```python
from build123d import *

# Parameters (mm, degrees)
SKETCH5_W               = 175.26
SKETCH5_H               = 137.414
SKETCH5_W_2             = 165.1
SKETCH5_H_2             = 127.254
BOSS_EXTRUDE2_DEPTH     = 43.18
SKETCH7_W               = 175.26
SKETCH7_H               = 137.414
BOSS_EXTRUDE4_DEPTH     = 10.16
SKETCH9_W               = 127.254
SKETCH9_H               = 2.159
CUT_EXTRUDE1_DEPTH      = 8.128
CUT_EXTRUDE2_DEPTH      = 13.208
CUT_EXTRUDE2_DEPTH_BACK = 147.066
SKETCH11_W              = 88.9
SKETCH11_H              = 33.02
CUT_EXTRUDE3_DEPTH      = 10.16
SKETCH12_W              = 25.4
SKETCH12_H              = 25.4
BOSS_EXTRUDE5_DEPTH     = 76.2
SKETCH13_W              = 20.32
SKETCH13_H              = 20.32
CUT_EXTRUDE4_DEPTH      = 76.2
SKETCH14_R              = 2.54
BOSS_EXTRUDE6_DEPTH     = 7.62
SKETCH15_R              = 2.54
BOSS_EXTRUDE7_DEPTH     = 25.4


with BuildPart() as part:
    # Sketch5 → Boss-Extrude2 (new body)
    with BuildSketch(Plane(origin=(0, 0, 0), x_dir=(1, 0, 0), z_dir=(0, 1, 0))):
        with Locations((82.55, 63.627)):
            Rectangle(SKETCH5_W, SKETCH5_H)
        with Locations((82.55, 63.627)):
            Rectangle(SKETCH5_W_2, SKETCH5_H_2, mode=Mode.SUBTRACT)
    extrude(amount=BOSS_EXTRUDE2_DEPTH)

    # Sketch7 → Boss-Extrude4 (add)
    with BuildSketch(Plane(origin=(0, 0, 0), x_dir=(1, 0, 0), z_dir=(0, 1, 0))):
        with Locations((82.55, 63.627)):
            Rectangle(SKETCH7_W, SKETCH7_H)
    extrude(amount=-BOSS_EXTRUDE4_DEPTH)

    # Sketch9 → Cut-Extrude1 (cut)
    with BuildSketch(Plane(origin=(170.18, 0, 0), x_dir=(0, 0, -1), z_dir=(1, 0, 0))):
        with Locations((63.627, 1.0795)):
            Rectangle(SKETCH9_W, SKETCH9_H)
    extrude(amount=-CUT_EXTRUDE1_DEPTH, mode=Mode.SUBTRACT)

    # Sketch10 → Cut-Extrude2 (cut, two sides: drawn at the far end of the back side and taken through both)
    with BuildSketch(Plane.XY.offset(5.08).offset(-CUT_EXTRUDE2_DEPTH_BACK)):
        with BuildLine():
            Line((69.85, 43.18), (95.25, 43.18))
            Line((95.25, 43.18), (95.25, 7.62))
            ThreePointArc((95.25, 7.62), (93.018153673, 2.231846327), (87.63, 0))
            Line((87.63, 0), (77.47, 0))
            ThreePointArc((77.47, 0), (72.081846327, 2.231846327), (69.85, 7.62))
            Line((69.85, 7.62), (69.85, 43.18))
        make_face()
    extrude(amount=CUT_EXTRUDE2_DEPTH + CUT_EXTRUDE2_DEPTH_BACK, mode=Mode.SUBTRACT)

    # Sketch11 → Cut-Extrude3 (cut)
    with BuildSketch(Plane.XZ.offset(10.16)):
        with Locations((82.55, -63.627)):
            Rectangle(SKETCH11_W, SKETCH11_H)
    extrude(amount=-CUT_EXTRUDE3_DEPTH, mode=Mode.SUBTRACT)

    # Sketch12 → Boss-Extrude5 (add)
    with BuildSketch(Plane.XZ.offset(10.16)):
        with Locations((7.62, -7.62)):
            Rectangle(SKETCH12_W, SKETCH12_H)
        with Locations((157.48, -7.62)):
            Rectangle(SKETCH12_W, SKETCH12_H)
        with Locations((157.48, -119.634)):
            Rectangle(SKETCH12_W, SKETCH12_H)
        with Locations((7.62, -119.634)):
            Rectangle(SKETCH12_W, SKETCH12_H)
    extrude(amount=BOSS_EXTRUDE5_DEPTH)

    # Sketch13 → Cut-Extrude4 (cut)
    with BuildSketch(Plane.XZ.offset(86.36)):
        with Locations((7.62, -7.62)):
            Rectangle(SKETCH13_W, SKETCH13_H)
        with Locations((157.48, -7.62)):
            Rectangle(SKETCH13_W, SKETCH13_H)
        with Locations((157.48, -119.634)):
            Rectangle(SKETCH13_W, SKETCH13_H)
        with Locations((7.62, -119.634)):
            Rectangle(SKETCH13_W, SKETCH13_H)
    extrude(amount=-CUT_EXTRUDE4_DEPTH, mode=Mode.SUBTRACT)

    # Sketch14 → Boss-Extrude6 (add)
    with BuildSketch(Plane.XY.offset(5.08)):
        with BuildLine():
            Line((69.409163099, -10.16), (69.409163099, -35.56))
            ThreePointArc((69.409163099, -35.56), (82.55, -48.700836901), (95.690836901, -35.56))
            Line((95.690836901, -35.56), (95.690836901, -10.16))
            Line((95.690836901, -10.16), (69.409163099, -10.16))
        make_face()
        with Locations((82.55, -35.56)):
            Circle(SKETCH14_R, mode=Mode.SUBTRACT)
    boss_extrude6 = extrude(amount=-BOSS_EXTRUDE6_DEPTH)

    # Mirror2: Boss-Extrude6 across plane
    add(boss_extrude6.mirror(Plane.XY.offset(-63.627)))

    # Sketch15 → Boss-Extrude7 (add)
    with BuildSketch(Plane(origin=(0, 0, -132.334), x_dir=(-1, 0, 0), z_dir=(0, 0, -1))):
        with Locations(Location((-122.428, 13.97, 0), (0, 0, 180))):
            Circle(SKETCH15_R)
    extrude(amount=BOSS_EXTRUDE7_DEPTH)


solid = part.part
```
CAD build for the part. Positions are in the model's coordinates, mm. A direction names the side the tool comes from. Coordinates: 2 decimals unless noted, no trailing zeros. Write each loop counter-clockwise with the first axis right and the second up, starting at its lowest first coordinate (ties: lowest second). Pieces come first, ordered by that corner, then holes. Notation, with made-up numbers: (4.5, -15.75) -> (60.5, -15.75) arc R34 ccw to (60.5, 17.25) -> close; hole circle Ø7 at (69.5, -29). An arc over 180 degrees is marked (long way). Return JSON: item names as keys, results as strings. Group by question number.
Q1. Flat gauge pins, fed straight in: pin 1 (10 mm diameter, centred on x = 156, y = -49, fed in from -Z); pin 2 (12 mm diameter, centred on x = 61.5, z = -86, fed in from +Y); pin 3 (10 mm diameter, centred on x = 11.5, z = -123.5, fed in from -Y). Where does each tip first touch, or does it go through?
Q2. Cut at A-A, the plane y = -65. State how many separate pieces and enclosed holes the cut face has, then the cut area to 3 significant figures.
Q3. Drill centre lines: line 1 (X direction, y = -79, z = -10); line 2 (Z direction, x = 4.5, y = -57.5); line 3 (X direction, y = 10, z = -11.5). Where is each one in solid material? Low to high.
Q4. Cut at B-B, the plane x = 64. Give the cut face in (y, z), then the cut area to 3 significant figures.
Q5. Pull direction Z, two halves, no side cores. Call faces 1 (the face through (146, -86.36, -7)), 2 (the face through (7, -48, -106.934)): released by +Z, released by -Z, zero draft, split by the parting line, or undercut.
Q6. Cut at D-D, the plane z = -99. Give the cut face in (x, y), then the cut area to 3 significant figures.
Q7. Which spindle directions (+Z, -Z, +X, -X, +Y, -Y) get a long thin tool onto all of the face, cutting with end or side? Do faces 3 (the face through (157, -10.16, -119)), 4 (the face through (72.141, 2.173, 2.504)), 5 (the face through (168, 2.159, -63)), 6 (the face through (20.32, -48, -8)), 7 (the face through (127, -5, -64)). Say none if no direction does.
Q8. Cut at C-C, the plane y = 13.97. Give the cut face in (x, z), then the cut area to 3 significant figures.
Returned:
{
 "1": {"pin 1": "stops at z = -132.33", "pin 2": "stops at y = 0", "pin 3": "stops at y = -10.16"},
 "2": {"separate pieces": "4", "enclosed holes": "4", "area": "929 mm2"},
 "3": {"line 1": "x = -5.08 to -2.54, 17.78 to 20.32, 144.78 to 147.32, 167.64 to 170.18", "line 2": "z = -132.33 to -129.79, -109.47 to -106.93, -20.32 to -17.78, 2.54 to 5.08", "line 3": "x = -5.08 to 0, 165.1 to 170.18"},
 "4": {"outline": "(-10.16, -132.33) -> (43.18, -132.33) -> (43.18, -127.25) -> (0, -127.25) -> (0, -80.14) -> (-10.16, -80.14) -> close; (-10.16, -47.12) -> (0, -47.12) -> (0, 0) -> (43.18, 0) -> (43.18, 5.08) -> (-10.16, 5.08) -> close", "area": "1,500 mm2"},
 "5": {"face 1": "zero draft", "face 2": "undercut"},
 "6": {"outline": "(-5.08, -10.16) -> (170.18, -10.16) -> (170.18, 0) -> (0, 0) -> (0, 43.18) -> (-5.08, 43.18) -> close; (165.1, 2.16) -> (170.18, 2.16) -> (170.18, 43.18) -> (165.1, 43.18) -> close", "area": "2,210 mm2"},
 "7": {"face 3": "-Y", "face 4": "+Z, -Z, +Y", "face 5": "+X", "face 6": "+Z, -Z, -Y", "face 7": "+Y, -Y"},
 "8": {"outline": "(-5.08, -132.33) -> (69.85, -132.33) -> (69.85, -127.25) -> (0, -127.25) -> (0, 0) -> (69.85, 0) -> (69.85, 5.08) -> (-5.08, 5.08) -> close; (95.25, -132.33) -> (119.89, -132.33) -> (119.89, -157.73) -> (124.97, -157.73) -> (124.97, -132.33) -> (170.18, -132.33) -> (170.18, 5.08) -> (95.25, 5.08) -> (95.25, 0) -> (165.1, 0) -> (165.1, -127.25) -> (95.25, -127.25) -> close", "area": "2,940 mm2"}
}
